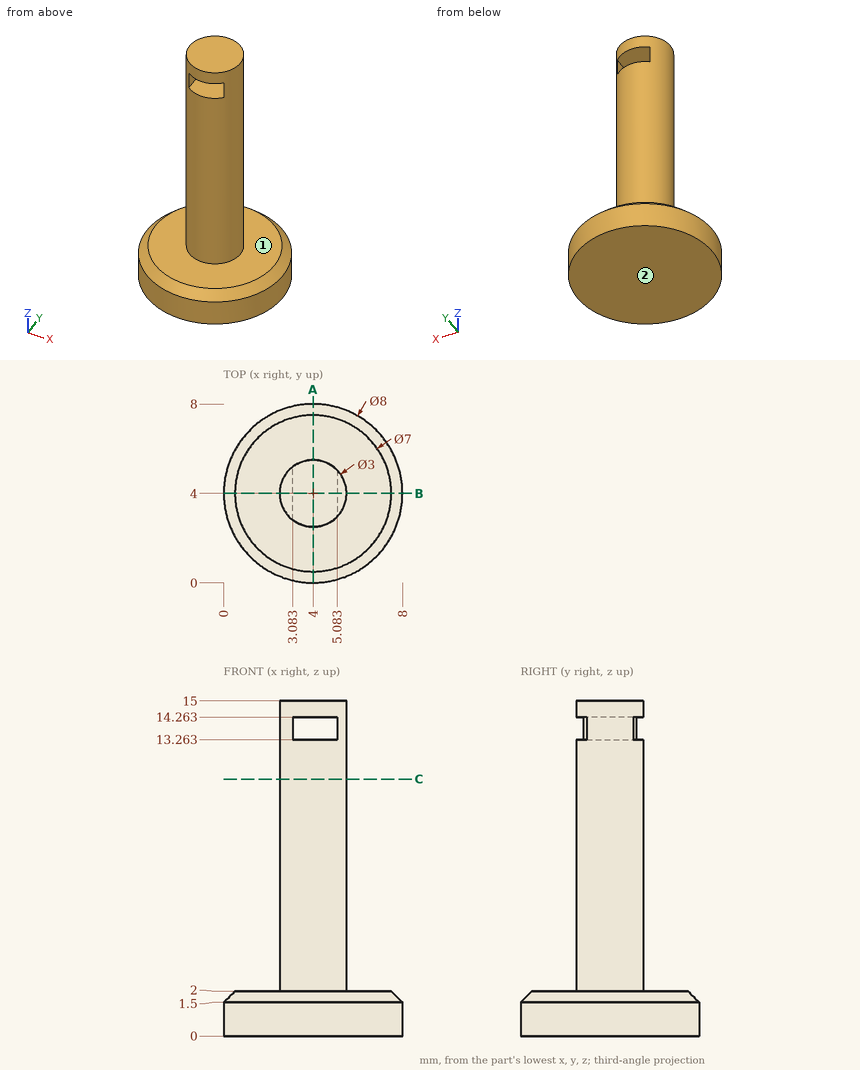
Source: three-view drawing plus pictorial views. Frame: mm from the lowest corner of the part. A direction names the side the tool comes from. Coordinates: 2 decimals unless noted, no trailing zeros. Order: outer loops, then holes, each group sorted by start corner. A loop starts at its lowest first (then second) coordinate and runs counter-clockwise, first axis right, second up.
Item 1: Cut plane A-A (x = 4). Return loops of the section in (y, z).
Output values:
outline: (0, 0) - (8, 0) - (8, 1.5) - (7.5, 2) - (5.5, 2) - (5.5, 13.26) - (2.5, 13.26) - (2.5, 2) - (0.5, 2) - (0, 1.5) - close; (2.5, 14.26) - (5.5, 14.26) - (5.5, 15) - (2.5, 15) - close
Item 2: First-contact query: P1, Ø1.1, axis at y = 4.5, z = 13.5, coming from the +X side; P2, Ø3, axis at x = 6.5, y = 1, coming from the +Z side; P3, Ø1.5, axis at y = 2.5, z = 13, coming from the +X side. Flat tips, straight axial feed; report the tip coordinate or a pass-through.
Output values:
P1: stops at x = 5.5
P2: stops at z = 2
P3: stops at x = 5.3
Item 3: Cut plane B-B (y = 4). Return loops of the section in (x, z).
Output values:
outline: (0, 0) - (8, 0) - (8, 1.5) - (7.5, 2) - (5.5, 2) - (5.5, 15) - (2.5, 15) - (2.5, 2) - (0.5, 2) - (0, 1.5) - close; hole (3.08, 13.26) - (5.08, 13.26) - (5.08, 14.26) - (3.08, 14.26) - close
Item 4: Cut plane C-C (z = 11.5). Return loops of the section in (x, y).
Output values:
outline: circle Ø3 at (4, 4)
Item 5: Material intervals for line 1 (Z direction, x = 3.25, y = 3.75); line 2 (Z direction, x = 3.5, y = 6.5); line 3 (Y direction, x = 4, z = 5.5), sorted ascending.
Output values:
line 1: z = 0 to 13.26, 14.26 to 15
line 2: z = 0 to 2
line 3: y = 2.5 to 5.5
Item 6: Set-up query: the marked faces 1 and 2. Return all of +Z, -Z, +X, -X, +Y, -Y with unobstructed straight access to the full face (end or side cutting, diameter ignored); none if empty.
Output values:
face 1: +Z
face 2: -Z, +X, -X, +Y, -Y
